Autodesk Inventor part; units mm, degrees
ref_plane "YZ Plane" through (0, 0, 0) normal (1, 0, 0) x (0, 1, 0)
ref_plane "XZ Plane" through (0, 0, 0) normal (0, 1, 0) x (-1, 0, 0)
ref_plane "XY Plane" through (0, 0, 0) normal (0, 0, 1) x (1, 0, 0)
sketch "Sketch1" plane through (0, 0, 0) normal (0, 0, 1) x (1, 0, 0)
  circle A0 centre (0, 0) radius 33.25
  circle A1 centre (0, 0) radius 26.475
  circle A2 centre (0, 0) radius 35.25
  dimension "d0" = 66.5
  dimension "d1" = 52.95
  dimension "d2" = 2
extrude "Extrusion1" add sketch "Sketch1" along normal blind 10.35
sketch "Sketch2" plane through (0, 0, 10.35) normal (0, 0, 1) x (1, 0, 0)
  circle A0 centre (0, 0) radius 35.25
extrude "Extrusion2" add sketch "Sketch2" against normal blind 0.5
sketch "Sketch3" plane through (0, 0, 10.35) normal (0, 0, 1) x (1, 0, 0)
  circle A0 centre (0, 0) radius 16
  dimension "d7" = 32
extrude "Extrusion3" cut sketch "Sketch3" against normal blind 2.5
sketch "Sketch4" plane through (0, 0, 7.85) normal (0, 0, 1) x (1, 0, 0)
  circle A0 centre (0, 0) radius 17.25
  dimension "d10" = 34.5
extrude "Extrusion4" cut sketch "Sketch4" against normal blind 3.1
sketch "Sketch5" plane through (0, 0, 4.75) normal (0, 0, 1) x (1, 0, 0)
  line L0 (-20.4, 17.85) -> (20.4, 17.85)
  line L1 (20.4, 17.85) -> (20.4, -17.85)
  line L2 (20.4, -17.85) -> (-20.4, -17.85)
  line L3 (-20.4, -17.85) -> (-20.4, 17.85)
  point P0 (0, 0)
  dimension "d13" = 40.8
  dimension "d14" = 35.7
  dimension "d15" = 17.85
  dimension "d16" = 20.4
extrude "Extrusion5" cut sketch "Sketch5" against normal through all
chamfer "Chamfer1" distance 0.8 angle 45 1 edges at (-16, 0, 10.35)
sketch "Sketch6" plane through (0, 0, 9.85) normal (0, 0, -1) x (-1, 0, 0)
  circle A0 centre (0, 0) radius 33.25
  circle A1 centre (0, 0) radius 26.475
extrude "Extrusion6" add sketch "Sketch6" along normal up to surface (5.1 mm away)
chamfer "Chamfer4" distance 1 angle 45 1 edges at (-16, 0, 7.85)
sketch "Sketch7" plane through (0, 0, 0) normal (0, 0, -1) x (-1, 0, 0)
  line L0 (8.9, -41.2726) -> (-1.1, -41.2726)
  line L1 (-1.1, -41.2726) -> (-1.1, 4.8372)
  line L2 (-1.1, 4.8372) -> (8.9, 4.8372)
  line L3 (8.9, 4.8372) -> (8.9, -41.2726)
  line L4 (19.5526, -17.85) -> (-19.5526, -17.85)
  line L5 (-20.4, -16.875) -> (-20.4, 16.875)
  line L6 (20.4, 16.875) -> (20.4, -16.875)
  point P0 (0, 0)
  point P1 (3.9, -41.2726)
  dimension "d36" = 10
  dimension "d40" = 21.5
extrude "Extrusion7" cut sketch "Sketch7" against normal up to surface (4.75 mm away)
sketch "Sketch8" plane through (0, 0, 10.35) normal (0, 0, 1) x (1, 0, 0)
  circle A0 centre (0, 0) radius 35.25
  circle A1 centre (0, 0) radius 28.25
  dimension "d41" = 7
extrude "Extrusion8" cut sketch "Sketch8" against normal blind 4.7
chamfer "Chamfer5" distance 8 angle 22 1 edges at (-28.25, 0, 10.35) measured on face at (23.997, -3.5937, 10.35)
chamfer "Chamfer6" distance 1.6 angle 45 1 edges at (-35.25, 0, 5.65)
chamfer "Chamfer7" distance 1.4 angle 45 1 edges at (-28.25, 0, 5.65)
properties part number "controls_knob_cover"
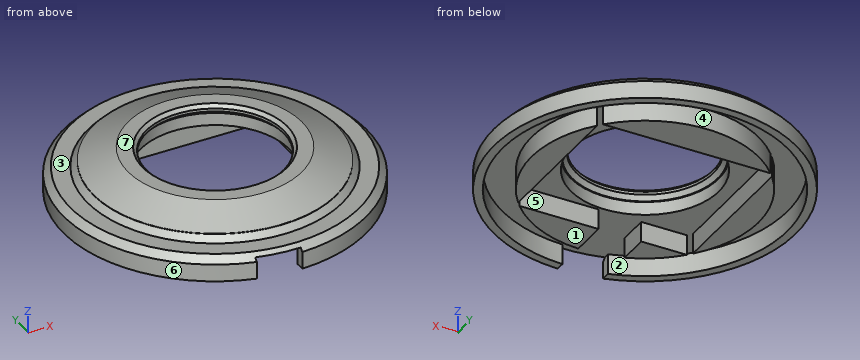
Geometry check sheet. Reference: the model listing, model coordinates, mm. Face numbers are marked on the shaded views. A direction names the side the tool comes from. Give positions to 0.01 mm unless a question says otherwise; leave off trailing zeros. Write each question's results on one line, items separated by ' | '. Start each with the question number.
(1) Gauge pin test, flat ends, axial feed: P1, Ø5, axis at y = -3, z = 1.5, coming from the -X side; P2, Ø1.4, axis at x = 9.5, z = 2.5, coming from the -Y side; P3, Ø4, axis at y = -22, z = 2, coming from the -X side. Record the tip position at first contact, or that the pin passes through.
(2) Mould release check, pull along X, two halves, no side actions. Record for the marked faces 4, 5, 6 and 7: pulls with the +X half, pulls with the -X half, needs draft (parallel to the pull), parting line crosses it, or undercut.
(3) Access from +Z, -Z, +X, -X, +Y, -Y to the whole of each face (thin tool, end or side, straight path). Record for the marked faces 1, 2 and 3.
(4) Scan lines: line 1 (X direction, y = 0, z = 3) (3 decimals); line 2 (X direction, y = -8, z = 2.75); line 3 (Y direction, x = 22, z = 2.5). Record each from-to range of solid material in increasing order.
Answer below:
1) P1: x = -35.25 | P2: y = -34.13 | P3: x = -29.03
2) face 4: undercut | face 5: undercut | face 6: parting line crosses it | face 7: needs draft
3) face 1: -Z, +X, -X, +Y, -Y | face 2: -Z | face 3: +Z
4) line 1: -35.25 to -33.25, -26.475 to -20.4, 20.4 to 26.475, 33.25 to 35.25 | line 2: -34.33 to -32.27, -25.24 to -20.4, 20.4 to 25.24, 32.27 to 34.33 | line 3: -27.54 to -24.93, -14.73 to 14.73, 24.93 to 27.54
